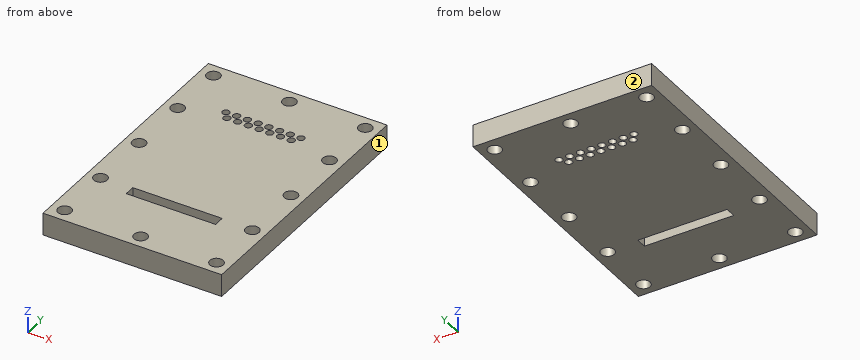
from build123d import *

# Parameters (mm, degrees)
F0_W     = 100
F0_H     = 150
F1_DEPTH = 12.5
F2_R     = 3.75
F3_DEPTH = 25
F4_W     = 50
F4_H     = 6
F5_DEPTH = 25
F6_R     = 2
F7_DEPTH = 25


# Not quite as in the source:
# - a feature names something its author has since deleted; it is built from what else it names


with BuildPart() as f1:
    # F0 (on Top) → F1 (new body)
    with BuildSketch(Plane.XY):
        Rectangle(F0_W, F0_H)
    extrude(amount=F1_DEPTH)

    # F2 (on face) → F3 (cut)
    with BuildSketch(Plane.XY.offset(12.5)):
        with Locations((-42.5, 67.5)):
            Circle(F2_R)
        with Locations((-42.5, 0)):
            Circle(F2_R)
        with Locations((-42.5, -35)):
            Circle(F2_R)
        with Locations((-42.5, -67.5)):
            Circle(F2_R)
        with Locations((0, -67.5)):
            Circle(F2_R)
        with Locations((-42.5, 35)):
            Circle(F2_R)
        with Locations((42.5, -67.5)):
            Circle(F2_R)
        with Locations((42.5, -35)):
            Circle(F2_R)
        with Locations((42.5, 0)):
            Circle(F2_R)
        with Locations((42.5, 35)):
            Circle(F2_R)
        with Locations((42.5, 67.5)):
            Circle(F2_R)
        with Locations((0, 67.5)):
            Circle(F2_R)
    extrude(amount=-F3_DEPTH, mode=Mode.SUBTRACT)

    # F4 (on face) → F5 (cut)
    with BuildSketch(Plane.XY.offset(12.5)):
        with Locations((0, -37)):
            Rectangle(F4_W, F4_H)
    extrude(amount=-F5_DEPTH, mode=Mode.SUBTRACT)

    # F6 (on face) → F7 (cut)
    with BuildSketch(Plane.XY.offset(12.5)):
        with Locations((-18, 40)):
            Circle(F6_R)
        with Locations((-15, 44)):
            Circle(F6_R)
        with Locations((-12, 40)):
            Circle(F6_R)
        with Locations((-9, 44)):
            Circle(F6_R)
        with Locations((-6, 40)):
            Circle(F6_R)
        with Locations((0, 40)):
            Circle(F6_R)
        with Locations((-3, 44)):
            Circle(F6_R)
        with Locations((-21, 44)):
            Circle(F6_R)
        with Locations((15, 44)):
            Circle(F6_R)
        with Locations((6, 40)):
            Circle(F6_R)
        with Locations((18, 40)):
            Circle(F6_R)
        with Locations((3, 44)):
            Circle(F6_R)
        with Locations((21, 44)):
            Circle(F6_R)
        with Locations((12, 40)):
            Circle(F6_R)
        with Locations((9, 44)):
            Circle(F6_R)
    extrude(amount=-F7_DEPTH, mode=Mode.SUBTRACT)


solid = f1.part
Input: part model. Units: mm. Frame: model coordinates. Face numbers are marked on the shaded views. Give positions to 0.01 mm unless a question says otherwise; leave off trailing zeros. Write each loop counter-clockwise with the first axis right and the second up, starting at its lowest first coordinate (ties: lowest second). Pieces come first, ordered by that corner, then holes. Notation, with made-up numbers: M -1.5,-39 L 40.5,-39 A23 cw 40.5,-18 Z; hole C 70.5,23.5 d1. An arc over 180 degrees is marked long. Write item = value, one per line. Start each with the question number.
1) Draft query along X for the marked faces 1 and 2. Return one class per face: +X half, -X half, draft (parallel to the pull), parting line (faces both ways), or undercut.
2) Cut plane A-A on y = 35. Return the cut outline in (x, z).
3) Cut plane C-C on z = 11. Count the separate pieces of the cut face and the enclosed holes in it, then the cut area to 3 significant figures.
4) Material intervals for line 1 along Y through (x, z) = (-12, 1.5); line 2 along Y through (x, z) = (0, 9.25); line 3 along Y through (x, z) = (-42.5, 5.5), sorted ascending. Write a range as [from, to].
5) Cut plane B-B on x = 42.5. Return the cut outline in (y, z), then the cut area to 3 significant figures.
Solved:
q1.face_1 = +X half
q1.face_2 = draft
q2.outline = M -50,0 L -46.25,0 L -46.25,12.5 L -50,12.5 Z; M -38.75,0 L 38.75,0 L 38.75,12.5 L -38.75,12.5 Z; M 46.25,0 L 50,0 L 50,12.5 L 46.25,12.5 Z
q3.separate_pieces = 1
q3.enclosed_holes = 28
q3.area = 14,000 mm2
q4.line_1 = [-75, -40], [-34, 38], [42, 75]
q4.line_2 = [-75, -71.25], [-63.75, -40], [-34, 38], [42, 63.75], [71.25, 75]
q4.line_3 = [-75, -71.25], [-63.75, -38.75], [-31.25, -3.75], [3.75, 31.25], [38.75, 63.75], [71.25, 75]
q5.outline = M -75,0 L -71.25,0 L -71.25,12.5 L -75,12.5 Z; M -63.75,0 L -38.75,0 L -38.75,12.5 L -63.75,12.5 Z; M -31.25,0 L -3.75,0 L -3.75,12.5 L -31.25,12.5 Z; M 3.75,0 L 31.25,0 L 31.25,12.5 L 3.75,12.5 Z; M 38.75,0 L 63.75,0 L 63.75,12.5 L 38.75,12.5 Z; M 71.25,0 L 75,0 L 75,12.5 L 71.25,12.5 Z
q5.area = 1,410 mm2
